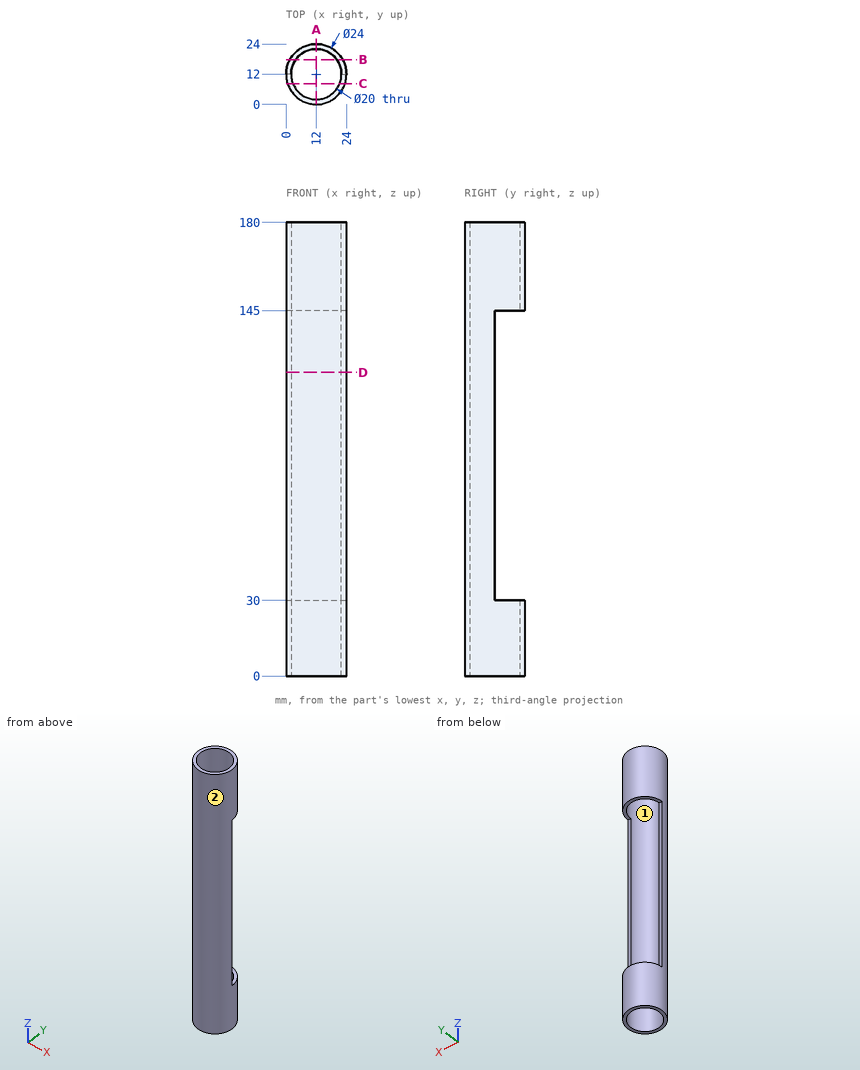
Here's the drawing with two shaded views (mm, measured from the low corner). I have some questions. Give positions to 0.01 mm unless a question says otherwise; leave off trailing zeros. Order: outer loops, then holes, each group sorted by start corner. A loop starts at its lowest first (then second) coordinate and runs counter-clockwise, first axis right, second up. Notation, with made-up numbers: (25.25, 57) -> (71.25, 57) arc R17 cw to (71.25, 82) -> close; hole circle Ø7 at (82.25, 64.25). An arc over 180 degrees is marked (long way). Use a Markdown table: item, result. Add a question column.
Item 1: Imagine slicing it at A-A on x = 12. Please give me the cut outline in (y, z), plus the area to 3 significant figures.
Item 2: Imagine slicing it at D-D on z = 120.5. Please give me the cut outline in (x, y).
Item 3: I need wall thicknesses on line 1 (Y direction, x = 11.25, z = 160.5); line 2 (Y direction, x = 12, z = 99); line 3 (Y direction, x = 3.5, z = 170). Which ranges of each line are inside material? Lowest first, please.
Item 4: Will these pins go through, and if not, where does the flat tip stop? pin 1 (2 mm diameter, centred on x = 23.5, z = 67, fed in from +Y); pin 2 (3 mm diameter, centred on y = 5, z = 24.5, fed in from -X); pin 3 (8 mm diameter, centred on y = 6, z = 73.5, fed in from -X).
Item 5: Imagine slicing it at C-C on y = 8.25. Please give me the cut outline in (x, z).
Item 6: If we mould it in two halves opening along X, with no side actions, what happens to the marked faces 1 and 2? For each: pulls with the +X half, pulls with the -X half, needs draft (parallel to the pull), parting line crosses it, or undercut.
Item 7: Imagine slicing it at B-B on y = 17.75. Please give me the cut outline in (x, z).
Data:
| question | item | result |
|---|---|---|
| 1 | outline | (0, 0) -> (2, 0) -> (2, 180) -> (0, 180) -> close; (22, 0) -> (24, 0) -> (24, 30) -> (22, 30) -> close; (22, 145) -> (24, 145) -> (24, 180) -> (22, 180) -> close |
| 1 | area | 490 mm² |
| 2 | outline | (0, 12) arc R12 ccw to (24, 12) -> (22, 12) arc R10 cw to (2, 12) -> close |
| 3 | line 1 | y = 0.02 to 2.03, 21.97 to 23.98 |
| 3 | line 2 | y = 0 to 2 |
| 3 | line 3 | y = 3.53 to 6.73, 17.27 to 20.47 |
| 4 | pin 1 | stops at y = 12 |
| 4 | pin 2 | stops at x = 1.33 |
| 4 | pin 3 | stops at x = 0.17 |
| 5 | outline | (0.6, 0) -> (2.73, 0) -> (2.73, 180) -> (0.6, 180) -> close; (21.27, 0) -> (23.4, 0) -> (23.4, 180) -> (21.27, 180) -> close |
| 6 | face 1 | undercut |
| 6 | face 2 | parting line crosses it |
| 7 | outline | (1.47, 0) -> (3.82, 0) -> (3.82, 30) -> (1.47, 30) -> close; (1.47, 145) -> (3.82, 145) -> (3.82, 180) -> (1.47, 180) -> close; (20.18, 0) -> (22.53, 0) -> (22.53, 30) -> (20.18, 30) -> close; (20.18, 145) -> (22.53, 145) -> (22.53, 180) -> (20.18, 180) -> close |
